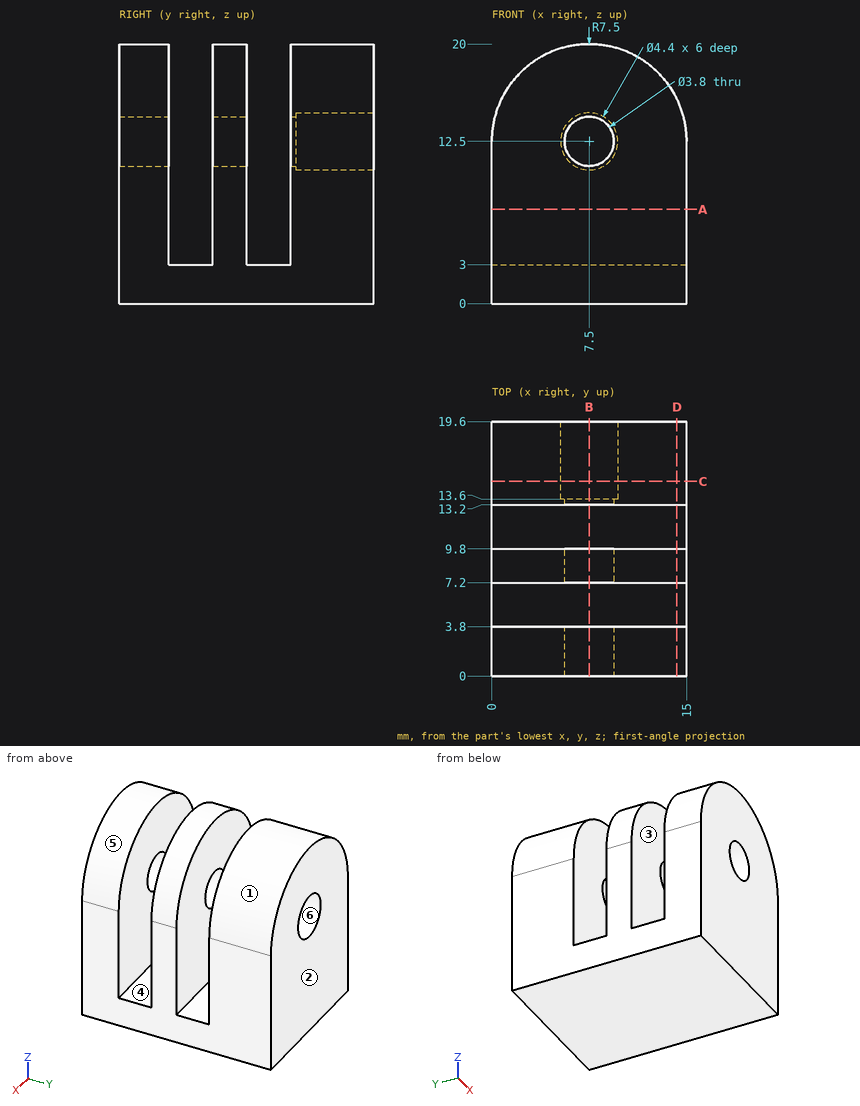
Geometry check sheet. Reference: drawing and pictorial views, mm from the part's lowest x, y, z. A direction names the side the tool comes from. Give positions to 0.01 mm unless a question says otherwise; leave off trailing zeros. Loops run counter-clockwise (first coordinate to the right, second up) from the corner with the lowest first, then second, coordinate; pieces in that order, holes last. Notation, with made-up numbers: M 16,26.25 L 36,26.25 A13 cw 36,35.25 Z; hole C -37.5,11 d8. An arc over 180 degrees is marked long. Use a Markdown table: item, result. Add a question column.
Q1. Scan lines: line 1 along Y through (x, z) = (2, 14.5); line 2 along Z through (x, y) = (7.5, 16.4); line 3 along Z through (x, y) = (7.5, 13.5). Record each from-to range of solid material in increasing order. Write a range as [from, to].
Q2. Sectioned sample at B-B, the plane x = 7.5. Record the cut outline in (y, z), then the cut area to 3 significant figures.
Q3. Tool access check on the marked faces 4, 5 and 6. Record the directions out of +Z, -Z, +X, -X, +Y, -Y that give a thin tool (end or side, any length) a straight path to the whole face; none if there is none.
Q4. Mould release check, pull along Y, two halves, no side actions. Record for the marked faces 1, 2 and 3: pulls with the +Y half, pulls with the -Y half, needs draft (parallel to the pull), parting line crosses it, or undercut.
Q5. Go/stop test with flat-tipped pins: pin 1 (2.5 mm diameter, centred on x = 4, y = 5.5, fed in from +Z); pin 2 (6 mm diameter, centred on y = 7, z = 12.5, fed in from -X); pin 3 (3.5 mm diameter, centred on x = 7.5, z = 12.5, fed in from +Y) (3 decimals); pin 4 (2 mm diameter, centred on x = 7.5, z = 11.5, fed in from +Y). Record where each tip stops, or that it passes through.
Q6. Sectioned sample at D-D, the plane x = 14.25. Record the cut outline in (y, z), then the cut area to 3 significant figures.
Q7. Sectioned sample at A-A, the plane z = 7.25. Record the cut outline in (x, y).
Q8. Sectioned sample at C-C, the plane y = 15. Record the cut outline in (x, z).
Verdict:
| question | item | result |
|---|---|---|
| 1 | line 1 | [0, 3.8], [7.2, 9.8], [13.2, 19.6] |
| 1 | line 2 | [0, 10.3], [14.7, 20] |
| 1 | line 3 | [0, 10.6], [14.4, 20] |
| 2 | outline | M 0,0 L 19.6,0 L 19.6,10.3 L 13.6,10.3 L 13.6,10.6 L 13.2,10.6 L 13.2,3 L 9.8,3 L 9.8,10.6 L 7.2,10.6 L 7.2,3 L 3.8,3 L 3.8,10.6 L 0,10.6 Z; M 0,14.4 L 3.8,14.4 L 3.8,20 L 0,20 Z; M 7.2,14.4 L 9.8,14.4 L 9.8,20 L 7.2,20 Z; M 13.2,14.4 L 13.6,14.4 L 13.6,14.7 L 19.6,14.7 L 19.6,20 L 13.2,20 Z |
| 2 | area | 224 mm^2 |
| 3 | face 4 | +Z, +X, -X |
| 3 | face 5 | +Z, +Y, -Y |
| 3 | face 6 | +Y |
| 4 | face 1 | needs draft |
| 4 | face 2 | pulls with the +Y half |
| 4 | face 3 | undercut |
| 5 | pin 1 | z = 3 |
| 5 | pin 2 | x = 0 |
| 5 | pin 3 | through |
| 5 | pin 4 | y = 13.6 |
| 6 | outline | M 0,0 L 19.6,0 L 19.6,15.77 L 13.2,15.77 L 13.2,3 L 9.8,3 L 9.8,15.77 L 7.2,15.77 L 7.2,3 L 3.8,3 L 3.8,15.77 L 0,15.77 Z |
| 6 | area | 222 mm^2 |
| 7 | outline | M 0,0 L 15,0 L 15,3.8 L 0,3.8 Z; M 0,7.2 L 15,7.2 L 15,9.8 L 0,9.8 Z; M 0,13.2 L 15,13.2 L 15,19.6 L 0,19.6 Z |
| 8 | outline | M 0,0 L 15,0 L 15,12.5 A7.5 ccw 0,12.5 Z; hole C 7.5,12.5 d4.4 |
